Source: CAD feature listing. Evaluate the final solid. Frame: model axes, mm. Give positions to 0.01 mm unless a question says otherwise; leave off trailing zeros. Order: outer loops, then holes, each group sorted by start corner. A loop starts at its lowest first (then second) coordinate and runs counter-clockwise, first axis right, second up. Notation, with made-up numbers: M 78.5,-31.5 L 101.5,-31.5 A14 ccw 101.5,-20.5 Z; hole C 25.5,74.25 d5. An arc over 180 degrees is marked long. Answer as a JSON object with one key per item and string values. Group by question number.
1. Section query C-C (z = -34). Output: boundary loops of the cut face in (x, y), plus the area to 3 significant figures.
2. Material intervals for L1, parallel to Z at x = -2.5, y = 5.5; L2, parallel to Y at x = 0, z = -78.65; L3, parallel to Y at x = 78.65, z = 0, sorted ascending. Write a range as [from, to].
3. Pull-direction query (Y, two-part tool) for faces 1 (the cylindrical face through (1.707, 14.568, 77.777)), 2 (the flat face through (-71, 0, -30)), 3 (the flat face through (-71, 25.4, -30)); classes: +Y half, -Y half, draft (parallel to the pull), parting line (faces both ways), or undercut.
4. Section query A-A (x = 0). Output: boundary loops of the cut face in (y, z) (3 decimals), plus the area to 3 significant figures.
5. Pin query (flat end, axial travel): P1, Ø3, axis at x = 51.5, y = 18, coming from the +Z side; P2, Ø5, axis at x = -34.5, y = 19.5, coming from the +Z side; P3, Ø6, axis at y = 23, z = 9, coming from the +X side; P4, Ø4, axis at x = 0, y = 11.89, coming from the -Z side. Return the tip coordinate at first contact, or that it passes through.
6. Section query B-B (z = 0). Output: boundary loops of the cut face in (x, y) (3 decimals).
7. Section query D-D (x = -32). Output: boundary loops of the cut face in (y, z).
from build123d import *

# Parameters (mm, degrees)
SKETCH1_R               = 79.375
SKETCH1_R_2             = 76.2
BOSS_EXTRUDE1_DEPTH     = 25.4
CUT_EXTRUDE4_START      = -3.210064
SKETCH2_R               = 2.3114
CUT_EXTRUDE4_DEPTH      = 3.210064
CIRPATTERN1_COUNT       = 4
SKETCH4_R               = 3.175
CUT_EXTRUDE6_DEPTH      = 1.000000113
CUT_EXTRUDE6_DEPTH_BACK = 159.750000113


with BuildPart() as part:
    # Sketch1 → Boss-Extrude1 (new body)
    with BuildSketch(Plane(origin=(0, 0, 0), x_dir=(1, 0, 0), z_dir=(0, 1, 0))):
        Circle(SKETCH1_R)
        Circle(SKETCH1_R_2, mode=Mode.SUBTRACT)
    extrude(amount=BOSS_EXTRUDE1_DEPTH)

    # Sketch2 → Cut-Extrude4 (cut)
    with BuildSketch(Plane.XY.offset(79.375).offset(CUT_EXTRUDE4_START)):
        with Locations((0, 11.890925676)):
            Circle(SKETCH2_R)
    cut_extrude4 = extrude(amount=CUT_EXTRUDE4_DEPTH, mode=Mode.SUBTRACT)

    # CirPattern1: Cut-Extrude4 ×4 about axis
    cirpattern1_axis = Axis((0, 25.4, 0), (0, -1, 0))
    for i in range(1, CIRPATTERN1_COUNT):
        add(cut_extrude4.rotate(cirpattern1_axis, i * 360 / CIRPATTERN1_COUNT), mode=Mode.SUBTRACT)

    # Sketch4 → Cut-Extrude6 (cut, two sides)
    with BuildSketch(Plane.XY.offset(79.375)) as cut_extrude6_sk:
        with Locations((0, 11.890925676)):
            Circle(SKETCH4_R)
    extrude(amount=CUT_EXTRUDE6_DEPTH, mode=Mode.SUBTRACT)
    extrude(cut_extrude6_sk.sketch, amount=-CUT_EXTRUDE6_DEPTH_BACK, mode=Mode.SUBTRACT)


solid = part.part
Answer sheet:
{
 "1": {"outline": "M -71.72,0 L -68.19,0 L -68.19,25.4 L -71.72,25.4 Z; M 68.19,0 L 71.72,0 L 71.72,25.4 L 68.19,25.4 Z", "area": "179 mm^2"},
 "2": {"L1": "[-79.34, -76.16], [76.16, 79.34]", "L2": "[0, 8.72], [15.07, 25.4]", "L3": "[0, 9.58], [14.2, 25.4]"},
 "3": {"face 1": "undercut", "face 2": "-Y half", "face 3": "+Y half"},
 "4": {"outline": "M 0,-79.375 L 8.716,-79.375 L 8.716,-76.2 L 0,-76.2 Z; M 0,76.2 L 8.716,76.2 L 8.716,79.375 L 0,79.375 Z; M 15.066,-79.375 L 25.4,-79.375 L 25.4,-76.2 L 15.066,-76.2 Z; M 15.066,76.2 L 25.4,76.2 L 25.4,79.375 L 15.066,79.375 Z", "area": "121 mm^2"},
 "5": {"P1": "z = 61.65", "P2": "z = 72.64", "P3": "x = 79.15", "P4": "through"},
 "6": {"outline": "M -79.375,0 L -76.2,0 L -76.2,9.58 L -79.375,9.58 Z; M -79.375,14.202 L -76.2,14.202 L -76.2,25.4 L -79.375,25.4 Z; M 76.2,0 L 79.375,0 L 79.375,9.58 L 76.2,9.58 Z; M 76.2,14.202 L 79.375,14.202 L 79.375,25.4 L 76.2,25.4 Z"},
 "7": {"outline": "M 0,-72.64 L 25.4,-72.64 L 25.4,-69.16 L 0,-69.16 Z; M 0,69.16 L 25.4,69.16 L 25.4,72.64 L 0,72.64 Z"}
}
